```python
from build123d import *

# Parameters (mm, degrees)
BOSS_EXTRUDE1_DEPTH     = 37
SKETCH2_W               = 73
SKETCH2_H               = 22
CUT_EXTRUDE2_DEPTH      = 2
CHAMFER1_SIZE           = 2
CHAMFER2_SIZE           = 2
CHAMFER3_SIZE           = 2
CHAMFER4_SIZE           = 2
SKETCH3_W               = 20
SKETCH3_H               = 20
CUT_EXTRUDE4_DEPTH      = 8
CUT_EXTRUDE5_DEPTH      = 107.292050502
SKETCH6_R               = 5
CUT_EXTRUDE6_DEPTH      = 108.284668057
CUT_EXTRUDE7_DEPTH      = 21
CUT_EXTRUDE7_DEPTH_BACK = 2
SKETCH8_R               = 3


with BuildPart() as part:
    # Sketch1 → Boss-Extrude1 (new body)
    with BuildSketch(Plane.XY):
        with BuildLine():
            Line((85, 0), (-85, 0))
            Line((-85, 0), (-82, 11))
            Line((-82, 11), (-48, 11))
            ThreePointArc((-48, 11), (-44.464466094, 12.464466094), (-43, 16))
            Line((-43, 16), (-43, 54))
            Line((-43, 54), (-22, 54))
            Line((-22, 54), (-22, 41))
            Line((-22, 41), (-19, 41))
            ThreePointArc((-19, 41), (0, 22), (19, 41))
            Line((19, 41), (22, 41))
            Line((22, 41), (22, 54))
            Line((22, 54), (43, 54))
            Line((43, 54), (43, 16))
            ThreePointArc((43, 16), (44.464466094, 12.464466094), (48, 11))
            Line((48, 11), (82, 11))
            Line((82, 11), (85, 0))
        make_face()
    extrude(amount=BOSS_EXTRUDE1_DEPTH)

    # Sketch2 → Cut-Extrude2 (cut)
    with BuildSketch(Plane(origin=(0, 0, 0), x_dir=(1, 0, 0), z_dir=(0, 1, 0))):
        with Locations((-40.5, -18.5)):
            Rectangle(SKETCH2_W, SKETCH2_H)
        with Locations((40.5, -18.5)):
            Rectangle(SKETCH2_W, SKETCH2_H)
    extrude(amount=CUT_EXTRUDE2_DEPTH, mode=Mode.SUBTRACT)

    # Chamfer1
    chamfer1_edges = [part.edges().sort_by_distance(p)[0] for p in [
        (-77, 2, 18.5),
    ]]
    chamfer(chamfer1_edges, length=CHAMFER1_SIZE - 0.0001)  # a hair under: the kernel refuses the full size

    # Chamfer2
    chamfer2_edges = [part.edges().sort_by_distance(p)[0] for p in [
        (4, 2, 18.5),
    ]]
    chamfer(chamfer2_edges, length=CHAMFER2_SIZE - 0.0001)  # a hair under: the kernel refuses the full size

    # Chamfer3
    chamfer3_edges = [part.edges().sort_by_distance(p)[0] for p in [
        (-4, 2, 18.5),
    ]]
    chamfer(chamfer3_edges, length=CHAMFER3_SIZE - 0.0001)  # a hair under: the kernel refuses the full size

    # Chamfer4
    chamfer4_edges = [part.edges().sort_by_distance(p)[0] for p in [
        (77, 2, 18.5),
    ]]
    chamfer(chamfer4_edges, length=CHAMFER4_SIZE - 0.0001)  # a hair under: the kernel refuses the full size

    # Sketch3 → Cut-Extrude4 (cut)
    with BuildSketch(Plane(origin=(0, 0, 0), x_dir=(1, 0, 0), z_dir=(0, 1, 0))):
        with Locations((-31, -18.5)):
            Rectangle(SKETCH3_W, SKETCH3_H)
        with Locations((31, -18.5)):
            Rectangle(SKETCH3_W, SKETCH3_H)
    extrude(amount=CUT_EXTRUDE4_DEPTH, mode=Mode.SUBTRACT)

    # Sketch5 → Cut-Extrude5 (cut, through all)
    with BuildSketch(Plane.XZ.offset(-2)):
        with BuildLine():
            Line((70, 23.582105154), (64, 23.582105154))
            ThreePointArc((64, 23.582105154), (59, 18.582105154), (64, 13.582105154))
            Line((64, 13.582105154), (70, 13.582105154))
            ThreePointArc((70, 13.582105154), (75, 18.582105154), (70, 23.582105154))
        make_face()
        with BuildLine():
            Line((-70, 23.582105154), (-64, 23.582105154))
            ThreePointArc((-64, 23.582105154), (-59, 18.582105154), (-64, 13.582105154))
            Line((-64, 13.582105154), (-70, 13.582105154))
            ThreePointArc((-70, 13.582105154), (-75, 18.582105154), (-70, 23.582105154))
        make_face()
    extrude(amount=-CUT_EXTRUDE5_DEPTH, mode=Mode.SUBTRACT)

    # Sketch6 → Cut-Extrude6 (cut, through all)
    with BuildSketch(Plane(origin=(0, 54, 0), x_dir=(1, 0, 0), z_dir=(0, 1, 0))):
        with Locations(Location((-31, -18.5, 0), (0, 0, 270))):
            Circle(SKETCH6_R)
        with Locations(Location((31, -18.5, 0), (0, 0, 270))):
            Circle(SKETCH6_R)
    extrude(amount=-CUT_EXTRUDE6_DEPTH, mode=Mode.SUBTRACT)

    # Sketch8 → Cut-Extrude7 (cut, two sides: drawn at the far end of the back side and taken through both)
    with BuildSketch(Plane(origin=(0, 16, 0), x_dir=(1, 0, 0), z_dir=(0, 1, 0)).offset(-CUT_EXTRUDE7_DEPTH_BACK)):
        with Locations(Location((0, -18.5, 0), (0, 0, 270))):
            Circle(SKETCH8_R)
    extrude(amount=CUT_EXTRUDE7_DEPTH + CUT_EXTRUDE7_DEPTH_BACK, mode=Mode.SUBTRACT)


solid = part.part
```
Work out the finished part from the listing and answer in its coordinate system (mm). A direction names the side the tool comes from. Give positions to 0.01 mm unless a question says otherwise; leave off trailing zeros. Loops run counter-clockwise (first coordinate to the right, second up) from the corner with the lowest first, then second, coordinate; pieces in that order, holes last. Notation, with made-up numbers: (-32.5, 28.5) -> (-2.5, 28.5) arc R25 ccw to (-2.5, 45.5) -> close; hole circle Ø8 at (74.5, 32.5). An arc over 180 degrees is marked (long way). Put each result on its own line as item: value. Start each with the question number.
Item 1: The mould has two halves that part along X. Classify faces 6 (the face through (26.12, 31.32, 17.42)), 7 (the face through (1, 0, 18)), 8 (the face through (83.48, 5.58, 18.24)): released by +X, released by -X, zero draft, split by the parting line, or undercut.
Item 2: Which of the six approach directions +Z, -Z, +X, -X, +Y, -Y give full straight-line access (tool end or side, diameter ignored) to faces 1 (the face through (-1.8, 18.1, 16.1)), 2 (the face through (26, 8, 16)), 3 (the face through (22, 47, 18)), 4 (the face through (1, 21, 0)), 5 (the face through (75, 6.4, 18.5))?
Item 3: Find the intervals of material crossed by L1, parallel to X at y = 40, z = 18; L2, parallel to X at y = 16, z = 18.5; L3, parallel to X at y = 49.5, z = 4.5, in increasing order. Write a range as [from, to].
Item 4: The part is cut by section D-D (y = 29). Give the vertices of the cut face in (x, z).
Item 5: The part is cut by section A-A (y = 45). Give the vertices of the cut face in (x, z).
Item 6: The part is cut by section B-B (x = -31). Give the vertices of the cut face in (y, z), then the cut area to 3 significant figures.
Item 7: The part is cut by section C-C (z = 5). Give the vertices of the cut face in (x, y).
Item 8: Each of these flat-tipped pins is pushed along its axis until it touches: P1, Ø6.5, axis at x = -46.5, z = 20, coming from the -Y side; P2, Ø10, axis at y = 32, z = 33, coming from the +X side; P3, Ø2.5, axis at x = 20.5, z = 25, coming from the +Y side; P4, Ø6, axis at x = -31, z = 18.5, coming from the -Y side. Where does it stop, or does it pass through?
Answers below:
1. face 6: undercut
1. face 7: zero draft
1. face 8: released by +X
2. face 1: +Y
2. face 2: -Y
2. face 3: +Z, -Z, +Y
2. face 4: -Z, +X, -X, +Y, -Y
2. face 5: +Y, -Y
3. L1: [-43, -35.97], [-26.03, -18.97], [18.97, 26.03], [35.97, 43]
3. L2: [-43, -36], [-26, -3], [3, 26], [36, 43]
3. L3: [-43, -22], [22, 43]
4. outline: (-43, 0) -> (-14.73, 0) -> (-14.73, 37) -> (-43, 37) -> close; (14.73, 0) -> (43, 0) -> (43, 37) -> (14.73, 37) -> close; hole circle Ø10 at (-31, 18.5); hole circle Ø10 at (31, 18.5)
5. outline: (-43, 0) -> (-22, 0) -> (-22, 37) -> (-43, 37) -> close; (22, 0) -> (43, 0) -> (43, 37) -> (22, 37) -> close; hole circle Ø10 at (-31, 18.5); hole circle Ø10 at (31, 18.5)
6. outline: (0, 0) -> (54, 0) -> (54, 13.5) -> (8, 13.5) -> (8, 8.5) -> (2, 8.5) -> (2, 7.5) -> (0, 7.5) -> close; (0, 29.5) -> (2, 29.5) -> (2, 28.5) -> (8, 28.5) -> (8, 23.5) -> (54, 23.5) -> (54, 37) -> (0, 37) -> close
6. area: 1,370 mm2
7. outline: (-85, 0) -> (85, 0) -> (82, 11) -> (48, 11) arc R5 cw to (43, 16) -> (43, 54) -> (22, 54) -> (22, 41) -> (19, 41) arc R19 cw to (-19, 41) -> (-22, 41) -> (-22, 54) -> (-43, 54) -> (-43, 16) arc R5 cw to (-48, 11) -> (-82, 11) -> close
8. P1: y = 2
8. P2: x = 43
8. P3: y = 41
8. P4: through
